Read the model definition and answer for the solid it produces. Units are mm, in the model's axes. Face numbers are marked on the shaded views. Give positions to 0.01 mm unless a question says otherwise; leave off trailing zeros. Write each loop counter-clockwise with the first axis right and the second up, starting at its lowest first coordinate (ties: lowest second). Pieces come first, ordered by that corner, then holes. Notation, with made-up numbers: (37.25, 75) -> (57.25, 75) arc R17 cw to (57.25, 99) -> close; hole circle Ø7 at (20.25, -15). An arc over 180 degrees is marked (long way). Answer as CSV lines item,"result". Start each with the question number.
1. The part is cut by section C-C, the plane y = -2. Determine the outline of the cut face in (x, z) (1 decimal), and give its area (3 significant figures).
2. Given pin 1 (7 mm diameter, centred on y = -2, z = -7.5, fed in from -X); pin 2 (8.5 mm diameter, centred on x = 0, z = 0, fed in from +Y); pin 3 (1.9 mm diameter, centred on x = -2.5, y = -3, fed in from +Z); pin 4 (10.5 mm diameter, centred on x = 0, z = 31.99, fed in from +Y) (3 decimals), each flat-ended and moving along its own axis, determine where each tip first touches the part or whether it passes through.
3. For a pull along X with two mould halves and no side action, classify the marked faces 1, 2 and 3 as pulls with the +X half, pulls with the -X half, needs draft (parallel to the pull), parting line crosses it, or undercut.
4. Find the intervals of material crossed by line 1 (Z direction, x = 0, y = -9.5) (3 decimals); line 2 (Y direction, x = 10.5, z = 7); line 3 (Z direction, x = 39, y = -2.25) (3 decimals), in increasing order.
5. The part is cut by section D-D, the plane x = -13. Determine the outline of the cut face in (y, z) (3 decimals).
6. The part is cut by section A-A, the plane z = 0. Determine the outline of the cut face in (x, y) (3 decimals), and give its area (3 significant figures).
7. The part is cut by section B-B, the plane x = 0.5. Determine the outline of the cut face in (y, z) (3 decimals), and give its area (3 significant figures).
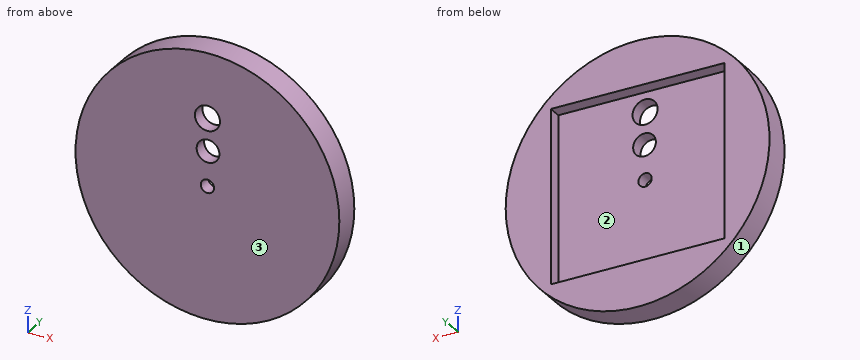
from build123d import *

# Parameters (mm, degrees)
F0_R     = 62.70625
F0_W     = 82.55
F0_H     = 82.55
F1_DEPTH = 12.7
F0_R_2   = 3.175
F0_R_3   = 5.401743
F0_R_4   = 5.953125
F2_DEPTH = 12.7
F3_DEPTH = 6.35


with BuildPart() as f1:
    # F0 (on Front) → F1 (new body)
    with BuildSketch(Plane.XZ):
        Circle(F0_R)
        Rectangle(F0_W, F0_H, mode=Mode.SUBTRACT)
    extrude(amount=F1_DEPTH)

    # F0 (on Front) → F2 (join)
    with BuildSketch(Plane.XZ):
        Rectangle(F0_W, F0_H)
        Circle(F0_R_2, mode=Mode.SUBTRACT)
        with Locations((0.268197, 16.59989)):
            Circle(F0_R_3, mode=Mode.SUBTRACT)
        with Locations((0, 31.988421)):
            Circle(F0_R_4, mode=Mode.SUBTRACT)
    extrude(amount=F2_DEPTH)

    # F0 (on Front) → F3 (cut)
    with BuildSketch(Plane.XZ):
        Rectangle(F0_W, F0_H)
        Circle(F0_R_2, mode=Mode.SUBTRACT)
        with Locations((0.268197, 16.59989)):
            Circle(F0_R_3, mode=Mode.SUBTRACT)
        with Locations((0, 31.988421)):
            Circle(F0_R_4, mode=Mode.SUBTRACT)
    extrude(amount=F3_DEPTH, mode=Mode.SUBTRACT)


solid = f1.part
Results found:
1,outline,"circle Ø125.4 at (0, 0); hole (-41.3, -41.3) -> (41.3, -41.3) -> (41.3, 41.3) -> (-41.3, 41.3) -> close"
1,area,"5,540 mm²"
2,pin 1,"stops at x = -62.58"
2,pin 2,"stops at y = -6.35"
2,pin 3,"stops at z = 62.69"
2,pin 4,"passes through"
3,face 1,"parting line crosses it"
3,face 2,"undercut"
3,face 3,"needs draft"
4,line 1,"z = -62.706 to -3.175, 3.175 to 11.205, 21.995 to 26.035, 37.942 to 62.706"
4,line 2,"y = -12.7 to -6.35"
4,line 3,"z = -49.103 to -41.275, 41.275 to 49.103"
5,outline,"(-12.7, -61.344) -> (0, -61.344) -> (0, -41.275) -> (-6.35, -41.275) -> (-6.35, 41.275) -> (0, 41.275) -> (0, 61.344) -> (-12.7, 61.344) -> close"
6,outline,"(-62.706, -12.7) -> (-3.175, -12.7) -> (-3.175, -6.35) -> (-41.275, -6.35) -> (-41.275, 0) -> (-62.706, 0) -> close; (3.175, -12.7) -> (62.706, -12.7) -> (62.706, 0) -> (41.275, 0) -> (41.275, -6.35) -> (3.175, -6.35) -> close"
6,area,"1,030 mm²"
7,outline,"(-12.7, -62.704) -> (0, -62.704) -> (0, -41.275) -> (-6.35, -41.275) -> (-6.35, -3.135) -> (-12.7, -3.135) -> close; (-12.7, 3.135) -> (-6.35, 3.135) -> (-6.35, 11.203) -> (-12.7, 11.203) -> close; (-12.7, 21.997) -> (-6.35, 21.997) -> (-6.35, 26.056) -> (-12.7, 26.056) -> close; (-12.7, 37.921) -> (-6.35, 37.921) -> (-6.35, 41.275) -> (0, 41.275) -> (0, 62.704) -> (-12.7, 62.704) -> close"
7,area,"885 mm²"
